Geometry: final body of the model. Coordinates: model frame, mm. Face numbers are marked on the shaded views. A direction names the side the tool comes from. Coordinates: 2 decimals unless noted, no trailing zeros. Write each loop counter-clockwise with the first axis right and the second up, starting at its lowest first coordinate (ties: lowest second). Pieces come first, ordered by that corner, then holes.
from build123d import *

# Parameters (mm, degrees)
F1_DEPTH = 14
F2_T     = -2.5
F4_DEPTH = 2.5


with BuildPart() as f1:
    # F0 (on Top) → F1 (new body)
    with BuildSketch(Plane.XY):
        with BuildLine():
            ThreePointArc((-9.6649585424, 8.357251808), (-22.1649585424, -4.142748192), (-9.6649585424, -16.642748192))
            Line((-9.6649585424, -16.642748192), (25.3350414576, -16.642748192))
            ThreePointArc((25.3350414576, -16.642748192), (37.8350414576, -4.142748192), (25.3350414576, 8.357251808))
            Line((25.3350414576, 8.357251808), (-9.6649585424, 8.357251808))
        make_face()
    extrude(amount=F1_DEPTH)

    # F2
    f2_openings = [f1.faces().sort_by_distance(p)[0] for p in [
        (7.835041, -4.142748, 14),
    ]]
    offset(amount=F2_T, openings=f2_openings)

    # F3 (on face) → F4 (join)
    with BuildSketch(Plane.XY.offset(14)):
        with BuildLine():
            ThreePointArc((25.3350414576, -16.642748192), (37.8350414576, -4.142748192), (25.3350414576, 8.357251808))
            Line((25.3350414576, 8.357251808), (-9.6649585424, 8.357251808))
            ThreePointArc((-9.6649585424, 8.357251808), (-22.1649585424, -4.142748192), (-9.6649585424, -16.642748192))
            Line((-9.6649585424, -16.642748192), (25.3350414576, -16.642748192))
        make_face()
        with BuildLine():
            Line((-9.6649585424, 7.107251808), (25.3350414576, 7.107251808))
            ThreePointArc((25.3350414576, 7.107251808), (36.5850414576, -4.142748192), (25.3350414576, -15.392748192))
            Line((25.3350414576, -15.392748192), (-9.6649585424, -15.392748192))
            ThreePointArc((-9.6649585424, -15.392748192), (-20.9149585424, -4.142748192), (-9.6649585424, 7.107251808))
        make_face(mode=Mode.SUBTRACT)
    extrude(amount=F4_DEPTH)


solid = f1.part
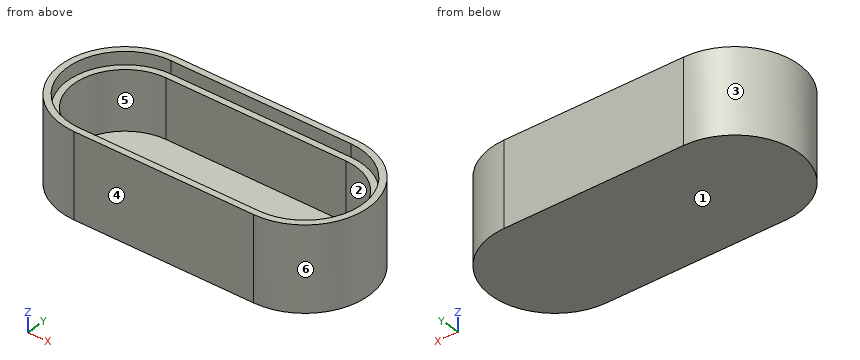
Item 1: Section A-A, the plane x = 1. Output: boundary loops of the cut face in (y, z).
Derived:
outline: (-16.64, 0) - (8.36, 0) - (8.36, 16.5) - (7.11, 16.5) - (7.11, 14) - (5.86, 14) - (5.86, 2.5) - (-14.14, 2.5) - (-14.14, 14) - (-15.39, 14) - (-15.39, 16.5) - (-16.64, 16.5) - close
Item 2: Pull-direction query (X, two-part tool) for the marked faces 3, 4, 5 and 6; classes: released by +X, released by -X, zero draft, split by the parting line, or undercut.
Derived:
face 3: released by -X
face 4: zero draft
face 5: undercut
face 6: released by +X
Item 3: Section C-C, the plane y = -8.75. Output: boundary loops of the cut face in (x, z) (3 decimals).
Derived:
outline: (-21.285, 0) - (36.955, 0) - (36.955, 16.5) - (35.598, 16.5) - (35.598, 14) - (34.21, 14) - (34.21, 2.5) - (-18.54, 2.5) - (-18.54, 14) - (-19.928, 14) - (-19.928, 16.5) - (-21.285, 16.5) - close
Item 4: Pin query (flat end, axial travel): pin 1 (1.5 mm diameter, centred on y = -2, z = 9.5, fed in from -X); pin 2 (3 mm diameter, centred on y = -9.5, z = 5, fed in from -X); pin 3 (10 mm diameter, centred on x = 7.5, y = -0.5, fed in from +Z). Return the tip coordinate at first contact, or that it passes through.
Derived:
pin 1: stops at x = -22.09
pin 2: stops at x = -21.55
pin 3: stops at z = 2.5
Item 5: Set-up query: the marked faces 1 and 2. Return all of +Z, -Z, +X, -X, +Y, -Y with unobstructed straight access to the full face (end or side cutting, diameter ignored); none if empty.
Derived:
face 1: -Z, +X, -X, +Y, -Y
face 2: +Z
Item 6: Material intervals for probe 1 along Y at (x, z) = (12, 11.25); probe 2 along Z at (x, y) = (-11.5, 0); probe 3 along X at (y, z) = (4, 11.5), sorted ascending.
Derived:
probe 1: y = -16.64 to -14.14, 5.86 to 8.36
probe 2: z = 0 to 2.5
probe 3: x = -19.15 to -15.47, 31.14 to 34.82
Item 7: Section B-B, the plane z = 8. Output: boundary loops of the cut face in (x, y), plus the area to 3 significant figures.
Derived:
outline: (-9.66, -16.64) - (25.34, -16.64) arc R12.5 ccw to (25.34, 8.36) - (-9.66, 8.36) arc R12.5 ccw to start; hole (-9.66, -14.14) - (25.34, -14.14) arc R10 ccw to (25.34, 5.86) - (-9.66, 5.86) arc R10 ccw to start
area: 352 mm2
